from build123d import *

# Parameters (mm, degrees)
CROQUIS2_W              = 200
CROQUIS2_H              = 155
CROQUIS2_W_2            = 31.297292299
CROQUIS2_H_2            = 43.768728426
CROQUIS2_H_3            = 43.768728427
CROQUIS2_W_3            = 23.573907934
CROQUIS2_H_4            = 45.323962431
SALIENTE_EXTRUIR1_DEPTH = 5
REDONDEO1_R             = 10
BOSS_EXTRUDE1_DEPTH     = 25
SKETCH3_W               = 62.040442094
SKETCH3_H               = 5.530821024
BOSS_EXTRUDE2_DEPTH     = 18
SKETCH8_W               = 62.040442094
SKETCH8_H               = 5.530821024
BOSS_EXTRUDE6_DEPTH     = 13


with BuildPart() as part:
    # Croquis2 → Saliente-Extruir1 (new body)
    with BuildSketch(Plane.XY):
        with Locations((0.108263467, -0.443414783)):
            Rectangle(CROQUIS2_W, CROQUIS2_H)
        with BuildLine():
            Line((-62.091736533, 71.556585217), (64.108263467, 71.556585217))
            ThreePointArc((64.108263467, 71.556585217), (67.108263467, 68.556585217), (64.108263467, 65.556585217))
            Line((64.108263467, 65.556585217), (-62.091736533, 65.556585217))
            ThreePointArc((-62.091736533, 65.556585217), (-65.091736533, 68.556585217), (-62.091736533, 71.556585217))
        make_face(mode=Mode.SUBTRACT)
        Polygon((-71.391736533, -12.98578064), (-71.391736533, 12.098951074), (-79.241736533, 12.123251884), (-83.891736533, 12.206585217), (-83.891736533, -13.093414783), (-79.241736533, -13.01008145), align=None, mode=Mode.SUBTRACT)
        with BuildLine():
            Line((92.108263467, 45.395048424), (92.108263467, -46.28187799))
            ThreePointArc((92.108263467, -46.28187799), (90.189031864, -47.362646387), (89.108263467, -45.443414783))
            Line((89.108263467, -45.443414783), (89.108263467, 44.556585217))
            ThreePointArc((89.108263467, 44.556585217), (90.189031864, 46.47581682), (92.108263467, 45.395048424))
        make_face(mode=Mode.SUBTRACT)
        Polygon((84.108263467, 12.206585217), (84.108263467, -13.093414783), (79.458263467, -13.093414783), (71.608263467, -13.093414783), (71.608263467, 12.206585217), (79.458263467, 12.206585217), align=None, mode=Mode.SUBTRACT)
        with BuildLine():
            Line((-91.891736533, 41.658521059), (-91.891736533, -42.545350625))
            ThreePointArc((-91.891736533, -42.545350625), (-90.590768612, -44.244382704), (-88.891736533, -42.943414783))
            Line((-88.891736533, -42.943414783), (-88.891736533, 42.056585217))
            ThreePointArc((-88.891736533, 42.056585217), (-90.590768612, 43.357553138), (-91.891736533, 41.658521059))
        make_face(mode=Mode.SUBTRACT)
        with Locations((-30.011405388, 36.299005811)):
            Rectangle(CROQUIS2_W_2, CROQUIS2_H_2, mode=Mode.SUBTRACT)
        with BuildLine():
            Line((-62.091736533, -72.443414783), (64.108263467, -72.443414783))
            ThreePointArc((64.108263467, -72.443414783), (67.108263467, -69.443414783), (64.108263467, -66.443414783))
            Line((64.108263467, -66.443414783), (-62.091736533, -66.443414783))
            ThreePointArc((-62.091736533, -66.443414783), (-65.091736533, -69.443414783), (-62.091736533, -72.443414783))
        make_face(mode=Mode.SUBTRACT)
        with Locations((-30.011405388, -26.799059535)):
            Rectangle(CROQUIS2_W_2, CROQUIS2_H_3, mode=Mode.SUBTRACT)
        with Locations((12.982877294, -0.693345879)):
            Rectangle(CROQUIS2_W_3, CROQUIS2_H_4, mode=Mode.SUBTRACT)
    extrude(amount=SALIENTE_EXTRUIR1_DEPTH)

    # Redondeo1
    redondeo1_edges = [part.edges().sort_by_distance(p)[0] for p in [
        (100.108263467, -77.943414783, 2.5),
        (-99.891736533, -77.943414783, 2.5),
        (-99.891736533, 77.056585217, 2.5),
        (100.108263467, 77.056585217, 2.5),
    ]]
    fillet(redondeo1_edges, radius=REDONDEO1_R)

    # Sketch1 → Boss-Extrude1 (add)
    with BuildSketch(Plane.XY.offset(5)):
        Polygon((-67.071845217, 64.976726992), (-67.071845217, 60.27797041), (-8.841198185, 60.27797041), (-8.841198185, 3.27797041), (-67.071845217, 3.27797041), (-67.071845217, 0.070097884), (-8.841198185, 0.070097884), (-8.841198185, -56.929902116), (-67.071845217, -56.929902116), (-67.071845217, -62.150742763), (-5.031403123, -62.150742763), (-5.031403123, -40.931443482), (46.608263467, -40.931443482), (46.608263467, -36.931443482), (-5.031403123, -36.931443482), (-5.031403123, 33.068556518), (46.608263467, 33.068556518), (46.608263467, 38.611481725), (-5.031403123, 38.611481725), (-5.031403123, 64.976726992), align=None)
    extrude(amount=BOSS_EXTRUDE1_DEPTH)

    # Sketch3 → Boss-Extrude2 (add)
    with BuildSketch(Plane.XZ.offset(62.150742763)):
        with Locations((-36.05162417, 27.234589488)):
            Rectangle(SKETCH3_W, SKETCH3_H)
    extrude(amount=BOSS_EXTRUDE2_DEPTH)

    # Sketch8 → Boss-Extrude6 (add)
    with BuildSketch(Plane(origin=(0, 64.976726992, 0), x_dir=(1, 0, 0), z_dir=(0, 1, 0))):
        with Locations((-36.05162417, -27.234589488)):
            Rectangle(SKETCH8_W, SKETCH8_H)
    extrude(amount=BOSS_EXTRUDE6_DEPTH)


solid = part.part
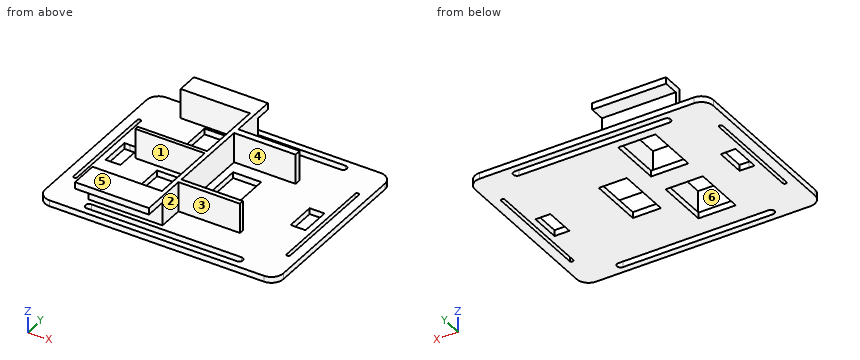
Could you check a few things on this model? Use its own coordinates, in mm. Face numbers are marked on the shaded views. A direction names the side the tool comes from. Give positions to 0.01 mm unless a question says otherwise; leave off trailing zeros. Order: outer loops, then holes, each group sorted by start corner. A loop starts at its lowest first (then second) coordinate and runs counter-clockwise, first axis right, second up.
1. Suppose I cut it at D-D (z = 27). List the corners of the cut face in (x, y) for me.
2. Suppose I cut it at C-C (y = -9). Give the number of separate pieces and of enclosed holes in the cut face, plus the area to 3 significant figures.
3. For the marked faces 4, 5 and 6, which set-ups out of +Z, -Z, +X, -X, +Y, -Y let a thin tool reach every point of the face, with its end or its side?
4. I need wall thicknesses on L1, parallel to Y at x = -12.5, z = 19.25; L2, parallel to X at y = 41, z = 2.25; L3, parallel to Y at x = 0.5, z = 4.5. Which ranges of each line are inside material? Lowest first, please.
5. Suppose I cut it at A-A (y = -29). List the corners of the cut face in (x, z) for me.
6. We'd pull the mould along Y, two halves only. Please class the marked faces 1, 2 and 3: pulls with the +Y half, pulls with the -Y half, needs draft (parallel to the pull), parting line crosses it, or undercut.
7. Will these pins go through, and if not, where does the flat tip stop? P1, Ø12, axis at y = 49.5, z = 20.5, coming from the +X side; P2, Ø1.5, axis at x = -22.5, z = 3.5, coming from the -Y side; P3, Ø9.5, axis at x = -46.5, z = 12.5, coming from the -Y side; P4, Ø5, axis at x = -22.5, y = -7.5, coming from the -Z side.
8. Suppose I cut it at B-B (x = 8). List the corners of the cut face in (y, z) for me, plus the area to 3 significant figures.
Solved:
1. outline: (-67.07, -80.15) - (-5.03, -80.15) - (-5.03, -40.93) - (46.61, -40.93) - (46.61, -36.93) - (-5.03, -36.93) - (-5.03, 33.07) - (46.61, 33.07) - (46.61, 38.61) - (-5.03, 38.61) - (-5.03, 77.98) - (-67.07, 77.98) - (-67.07, 60.28) - (-8.84, 60.28) - (-8.84, 3.28) - (-67.07, 3.28) - (-67.07, 0.07) - (-8.84, 0.07) - (-8.84, -56.93) - (-67.07, -56.93) - close
2. separate pieces: 7
2. enclosed holes: 0
2. area: 666 mm2
3. face 4: +Z, +X
3. face 5: +Z, +X, -X, +Y, -Y
3. face 6: +Z, -X
4. L1: y = -62.15 to -56.93, 0.07 to 3.28, 60.28 to 64.98
4. L2: x = -99.89 to -91.89, -88.89 to -45.66, -14.36 to 89.11, 92.11 to 100.11
4. L3: y = -77.94 to -72.44, -66.44 to 65.56, 71.56 to 77.06
5. outline: (-99.89, 0) - (-91.89, 0) - (-91.89, 5) - (-99.89, 5) - close; (-88.89, 0) - (-45.66, 0) - (-45.66, 5) - (-88.89, 5) - close; (-14.36, 0) - (89.11, 0) - (89.11, 5) - (-5.03, 5) - (-5.03, 30) - (-8.84, 30) - (-8.84, 5) - (-14.36, 5) - close; (92.11, 0) - (100.11, 0) - (100.11, 5) - (92.11, 5) - close
6. face 1: undercut
6. face 2: needs draft
6. face 3: pulls with the -Y half
7. P1: stops at x = -5.03
7. P2: stops at y = -77.94
7. P3: stops at y = -62.15
7. P4: passes through
8. outline: (-77.94, 0) - (-72.44, 0) - (-72.44, 5) - (-77.94, 5) - close; (-66.44, 0) - (-23.36, 0) - (-23.36, 5) - (-36.93, 5) - (-36.93, 30) - (-40.93, 30) - (-40.93, 5) - (-66.44, 5) - close; (21.97, 0) - (65.56, 0) - (65.56, 5) - (38.61, 5) - (38.61, 30) - (33.07, 30) - (33.07, 5) - (21.97, 5) - close; (71.56, 0) - (77.06, 0) - (77.06, 5) - (71.56, 5) - close
8. area: 727 mm2
